from build123d import *

# Parameters (mm, degrees)
F0_W     = 105.2859798074
F0_H     = 152.4502895772
F1_DEPTH = 34
F2_W     = 13.3893657476
F2_H     = 26.8833786249
F2_W_2   = 12.5688500702
F2_W_3   = 10.8668655157
F2_H_2   = 36.1870983616
F3_DEPTH = 51
F4_T     = -2.5


with BuildPart() as f1:
    # F0 (on Top) → F1 (new body)
    with BuildSketch(Plane.XY):
        with Locations((34.4720818102, 33.6500052363)):
            Rectangle(F0_W, F0_H)
    extrude(amount=F1_DEPTH)

    # F2 (on face) → F3 (join)
    with BuildSketch(Plane.XY.offset(34)):
        with Locations((6.6946828738, 84.6460089087)):
            Rectangle(F2_W, F2_H)
        with Locations((57.3803391308, 84.6460089087)):
            Rectangle(F2_W_2, F2_H)
        with Locations((37.0119139552, -5.1396149211)):
            Rectangle(F2_W_3, F2_H_2)
    extrude(amount=F3_DEPTH)

    # F4
    f4_openings = [f1.faces().sort_by_distance(p)[0] for p in [
        (37.011914, -5.139615, 85),
    ]]
    offset(amount=F4_T, openings=f4_openings, kind=Kind.INTERSECTION)


solid = f1.part
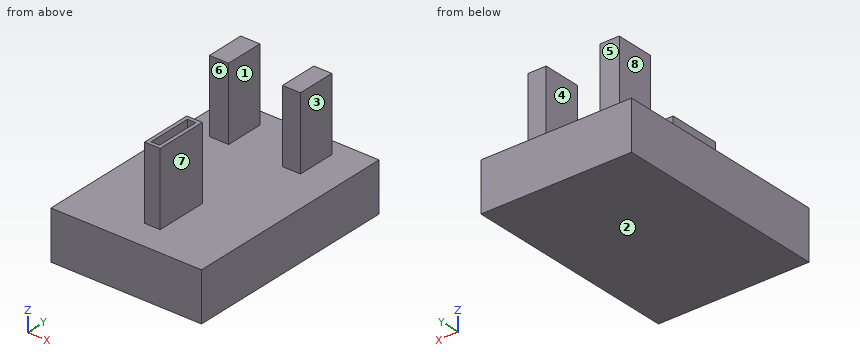
For this review, take the finished solid that the model builds, in its own axes (mm). Face numbers are marked on the shaded views. A direction names the side the tool comes from. Give positions to 0.01 mm unless a question says otherwise; leave off trailing zeros. Loops run counter-clockwise (first coordinate to the right, second up) from the corner with the lowest first, then second, coordinate; pieces in that order, holes last. Notation, with made-up numbers: M 16,26 L 39,26 A17 ccw 39,45 Z; hole C 53,35.5 d9. An arc over 180 degrees is marked long. Put each result on its own line as item: value. Start each with the question number.
(1) Machinability: for the marked faces 4, 5, 6, 7 and 8, which of the approach directions +Z, -Z, +X, -X, +Y, -Y give a long, thin tool a straight path to every point of the face, cutting with its end or side? Answer none if there is none.
(2) For pin 1 (18 mm diameter, centred on y = 3.5, z = 70, fed in from +X); pin 2 (5 mm diameter, centred on x = -2, z = 46, fed in from -Y); pin 3 (10 mm diameter, centred on x = 55.5, z = 54, fed in from +Y); pin 4 (1.5 mm diameter, centred on x = 16, z = 74, fed in from +Y), all flat-tipped, find the tip position at first contact; note any pin that passes through.
(3) Add section B-B, the plane y = 86.5. Write out the cut boundary in (x, z), then the cut area to 3 significant figures.
(4) Add section D-D, the plane x = 78.5. Write out the cut boundary in (y, z).
(5) Wall thickness on L1, parallel to X at y = 85.5, z = 37; L2, parallel to Y at x = -2, z = 19; L3, parallel to Z at x = 64.5, y = -20.5: over which ranges is each line inside the solid? List them lowest first.
(6) Add section C-C, the plane z = 28. Write out the cut boundary in (x, y).
(7) The part is to be moulded in two halves that separate along X. For the marked faces 1, 2 and 3, say which applies: +X half, -X half, draft (parallel to the pull), parting line (faces both ways), or undercut.
(8) Add section A-A, the plane z = 70.5. Write out the cut boundary in (x, y), then the cut area to 3 significant figures.
Result:
1. face 4: +Z, +Y, -Y
1. face 5: +Z, +X, -X, +Y
1. face 6: +Z, +X, -X, -Y
1. face 7: +Z, +X, +Y, -Y
1. face 8: +Z, -X, +Y, -Y
2. pin 1: stops at x = 42.45
2. pin 2: stops at y = 71.2
2. pin 3: stops at y = 98.09
2. pin 4: passes through
3. outline: M -18.17,0 L 87.12,0 L 87.12,34 L 63.66,34 L 63.66,85 L 51.1,85 L 51.1,34 L 13.39,34 L 13.39,85 L 0,85 L 0,34 L -18.17,34 Z; hole M -15.67,2.5 L 84.62,2.5 L 84.62,31.5 L 61.16,31.5 L 61.16,82.5 L 53.6,82.5 L 53.6,31.5 L 10.89,31.5 L 10.89,82.5 L 2.5,82.5 L 2.5,31.5 L -15.67,31.5 Z
3. area: 1,180 mm^2
4. outline: M -42.58,0 L 109.88,0 L 109.88,34 L -42.58,34 Z; hole M -40.08,2.5 L 107.38,2.5 L 107.38,31.5 L -40.08,31.5 Z
5. L1: x = 0 to 2.5, 10.89 to 13.39, 51.1 to 53.6, 61.16 to 63.66
5. L2: y = -42.58 to -40.08, 107.38 to 109.88
5. L3: z = 0 to 2.5, 31.5 to 34
6. outline: M -18.17,-42.58 L 87.12,-42.58 L 87.12,109.88 L -18.17,109.88 Z; hole M -15.67,-40.08 L 84.62,-40.08 L 84.62,107.38 L -15.67,107.38 Z
7. face 1: undercut
7. face 2: draft
7. face 3: +X half
8. outline: M 0,71.2 L 13.39,71.2 L 13.39,98.09 L 0,98.09 Z; M 31.58,-23.23 L 42.45,-23.23 L 42.45,12.95 L 31.58,12.95 Z; M 51.1,71.2 L 63.66,71.2 L 63.66,98.09 L 51.1,98.09 Z; hole M 2.5,73.7 L 10.89,73.7 L 10.89,95.59 L 2.5,95.59 Z; hole M 34.08,-20.73 L 39.95,-20.73 L 39.95,10.45 L 34.08,10.45 Z; hole M 53.6,73.7 L 61.16,73.7 L 61.16,95.59 L 53.6,95.59 Z
8. area: 559 mm^2
